```python
from build123d import *

# Parameters (mm, degrees)
EXTRUDE_1_DEPTH      = 55
CUT_EXTRUDE_START    = -5
SKETCH_2_R           = 18.75
SKETCH_2_R_2         = 14.75
CUT_EXTRUDE_1_DEPTH  = 59.016862823
EXTRUDE_3_REACH      = 65.017
EXTRUDE_3_END_RADIUS = 18.75
SKETCH_4_W           = 7
SKETCH_4_H           = 7
SKETCH_3_R           = 1.1
CUT_EXTRUDE_2_DEPTH  = 5
CUT_EXTRUDE_START_2  = -4
SKETCH_5_R           = 2.5
CUT_EXTRUDE_3_DEPTH  = 60.016862823
SKETCH_6_R           = 1.1
CUT_EXTRUDE_4_DEPTH  = 4


with BuildPart() as part:
    # ｽｹｯﾁ1 → ﾎﾞｽ - 押し出し1 (new body)
    with BuildSketch(Plane(origin=(0, 0, 0), x_dir=(1, 0, 0), z_dir=(0, 1, 0))):
        with BuildLine():
            Line((0, -21.75), (0, -14.75))
            ThreePointArc((0, -14.75), (-14.75, 0), (0, 14.75))
            Line((0, 14.75), (0, 21.75))
            ThreePointArc((0, 21.75), (-21.75, 0), (0, -21.75))
        make_face()
    extrude(amount=EXTRUDE_1_DEPTH)

    # ｽｹｯﾁ2 → ｶｯﾄ - 押し出し1 (cut, through all)
    with BuildSketch(Plane(origin=(0, 55, 0), x_dir=(1, 0, 0), z_dir=(0, 1, 0)).offset(CUT_EXTRUDE_START)):
        Circle(SKETCH_2_R)
        Circle(SKETCH_2_R_2, mode=Mode.SUBTRACT)
    extrude(amount=-CUT_EXTRUDE_1_DEPTH, mode=Mode.SUBTRACT)

    # ﾎﾞｽ - 押し出し3: up to this cylinder (the profile starts inside it)
    extrude_3_end = Plane(origin=(0, 25, 0), z_dir=(0, 1, 0)) * Cylinder(EXTRUDE_3_END_RADIUS, 193.534, mode=Mode.PRIVATE)
    # ｽｹｯﾁ4 → ﾎﾞｽ - 押し出し3 (add, up to the surface)
    with BuildSketch(Plane(origin=(0, 0, 0), x_dir=(0, 0, -1), z_dir=(1, 0, 0)), mode=Mode.PRIVATE) as extrude_3_sk1:
        with Locations((-18.25, 37.5)):
            Rectangle(SKETCH_4_W, SKETCH_4_H)
    extrude_3_tool1 = extrude(extrude_3_sk1.sketch, amount=-EXTRUDE_3_REACH, mode=Mode.PRIVATE) & extrude_3_end
    add(extrude_3_tool1.solids().sort_by_distance((0, 37.5, 18.25))[0])
    # ｽｹｯﾁ4 → ﾎﾞｽ - 押し出し3 (add, up to the surface)
    with BuildSketch(Plane(origin=(0, 0, 0), x_dir=(0, 0, -1), z_dir=(1, 0, 0)), mode=Mode.PRIVATE) as extrude_3_sk2:
        with Locations((-18.25, 12.5)):
            Rectangle(SKETCH_4_W, SKETCH_4_H)
    extrude_3_tool2 = extrude(extrude_3_sk2.sketch, amount=-EXTRUDE_3_REACH, mode=Mode.PRIVATE) & extrude_3_end
    add(extrude_3_tool2.solids().sort_by_distance((0, 12.5, 18.25))[0])
    # ｽｹｯﾁ4 → ﾎﾞｽ - 押し出し3 (add, up to the surface)
    with BuildSketch(Plane(origin=(0, 0, 0), x_dir=(0, 0, -1), z_dir=(1, 0, 0)), mode=Mode.PRIVATE) as extrude_3_sk3:
        with Locations((18.25, 12.5)):
            Rectangle(SKETCH_4_W, SKETCH_4_H)
    extrude_3_tool3 = extrude(extrude_3_sk3.sketch, amount=-EXTRUDE_3_REACH, mode=Mode.PRIVATE) & extrude_3_end
    add(extrude_3_tool3.solids().sort_by_distance((0, 12.5, -18.25))[0])
    # ｽｹｯﾁ4 → ﾎﾞｽ - 押し出し3 (add, up to the surface)
    with BuildSketch(Plane(origin=(0, 0, 0), x_dir=(0, 0, -1), z_dir=(1, 0, 0)), mode=Mode.PRIVATE) as extrude_3_sk4:
        with Locations((18.25, 37.5)):
            Rectangle(SKETCH_4_W, SKETCH_4_H)
    extrude_3_tool4 = extrude(extrude_3_sk4.sketch, amount=-EXTRUDE_3_REACH, mode=Mode.PRIVATE) & extrude_3_end
    add(extrude_3_tool4.solids().sort_by_distance((0, 37.5, -18.25))[0])

    # ｽｹｯﾁ3 → ｶｯﾄ - 押し出し2 (cut)
    with BuildSketch(Plane(origin=(0, 0, 0), x_dir=(0, 0, -1), z_dir=(1, 0, 0))):
        with Locations((-18.25, 37.5)):
            Circle(SKETCH_3_R)
        with Locations(Location((18.25, 37.5, 0), (0, 0, 180))):
            Circle(SKETCH_3_R)
        with Locations((18.25, 12.5)):
            Circle(SKETCH_3_R)
        with Locations(Location((-18.25, 12.5, 0), (0, 0, 180))):
            Circle(SKETCH_3_R)
    extrude(amount=-CUT_EXTRUDE_2_DEPTH, mode=Mode.SUBTRACT)

    # ｽｹｯﾁ5 → ｶｯﾄ - 押し出し3 (cut, through all)
    with BuildSketch(Plane(origin=(0, 0, 0), x_dir=(0, 0, -1), z_dir=(1, 0, 0)).offset(CUT_EXTRUDE_START_2)):
        with Locations((-18.25, 37.5)):
            Circle(SKETCH_5_R)
        with Locations((-18.25, 12.5)):
            Circle(SKETCH_5_R)
        with Locations((18.25, 12.5)):
            Circle(SKETCH_5_R)
        with Locations((18.25, 37.5)):
            Circle(SKETCH_5_R)
    extrude(amount=-CUT_EXTRUDE_3_DEPTH, mode=Mode.SUBTRACT)

    # ｽｹｯﾁ6 → ｶｯﾄ - 押し出し4 (cut)
    with BuildSketch(Plane(origin=(0, 55, 0), x_dir=(1, 0, 0), z_dir=(0, 1, 0))):
        with Locations(Location((-12.904698757, -12.904698757, 0), (0, 0, 270))):
            Circle(SKETCH_6_R)
        with Locations(Location((-12.904698757, 12.904698757, 0), (0, 0, 270))):
            Circle(SKETCH_6_R)
    extrude(amount=-CUT_EXTRUDE_4_DEPTH, mode=Mode.SUBTRACT)


solid = part.part
```
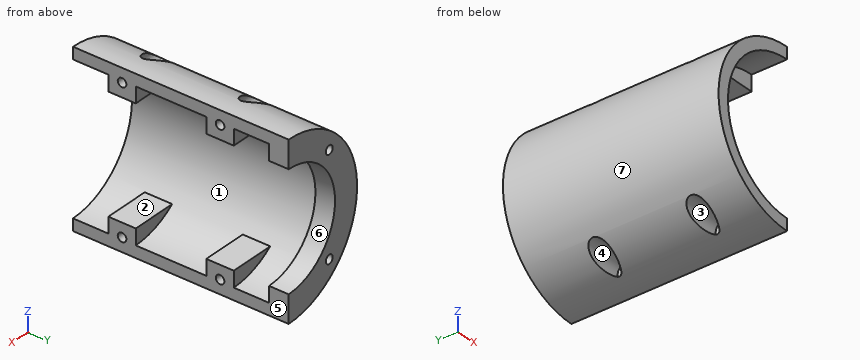
Check sheet for the modelled part. Datum: model origin and axes. Units: mm. Face numbers are marked on the shaded views. A direction names the side the tool comes from. Coordinates: 2 decimals unless noted, no trailing zeros. Write each loop counter-clockwise with the first axis right and the second up, starting at its lowest first coordinate (ties: lowest second). Pieces come first, ordered by that corner, then holes. Notation, with made-up numbers: (88, 9.5) - (128, 9.5) arc R29 ccw to (128, 39.5) - close; hole circle Ø3 at (-22, 46.5). An arc over 180 degrees is marked (long way). One line per question, with ' | ' between items.
Item 1: Sectioned sample at B-B on y = 37.5. Record the boundary of the cut face in (x, z).
Determined:
outline: (-15, -15.75) - (-4, -15.75) - (-4, -17.15) - (0, -17.15) - (0, -14.75) - (-11.58, -14.75) arc R18.75 cw to (-11.58, 14.75) - (0, 14.75) - (0, 17.15) - (-4, 17.15) - (-4, 15.75) - (-15, 15.75) arc R21.75 ccw to start; (-6.52, -20.75) arc R21.75 ccw to (0, -21.75) - (0, -19.35) - (-4, -19.35) - (-4, -20.75) - close; (-6.52, 20.75) - (-4, 20.75) - (-4, 19.35) - (0, 19.35) - (0, 21.75) arc R21.75 ccw to start
Item 2: Access from +Z, -Z, +X, -X, +Y, -Y to the whole of each face (thin tool, end or side, straight path). Record for the marked faces 1, 2 and 3.
Determined:
face 1: +X | face 2: +X, -Y | face 3: -X
Item 3: Gauge pin test, flat ends, axial feed: P1, Ø1.5, axis at x = -14.5, z = -2, coming from the -Y side; P2, Ø3, axis at x = -12.5, y = 32.5, coming from the +Z side; P3, Ø2, axis at y = 36, z = -4.5, coming from the +X side. Record the tip position at first contact, or that the pin passes through.
Determined:
P1: stops at y = 50 | P2: stops at z = 18.76 | P3: stops at x = -17.93
Item 4: Thickness scan on line 1 (Y direction, x = -1.15, z = -18.25); line 2 (Y direction, x = -6.25, z = 18.25); line 3 (Z direction, x = -5.25, y = 37.5). Record the ranges inside material, lowest first. Write a range as [from, to].
Determined:
line 1: y = [9, 11.4], [13.6, 16], [34, 36.4], [38.6, 41], [50, 55] | line 2: y = [0, 10], [15, 35], [40, 55] | line 3: z = [-21.11, -20.75], [-15.75, -14.75], [14.75, 15.75], [20.75, 21.11]
Item 5: Sectioned sample at A-A on x = -1.5. Give the number of separate pieces and of enclosed holes in the cut face, plus the area to 3 significant figures.
Determined:
separate pieces: 2 | enclosed holes: 4 | area: 466 mm2
Item 6: Sectioned sample at C-C on z = 0. Record the boundary of the cut face in (x, y), plus the area to 3 significant figures.
Determined:
outline: (-21.75, 0) - (-18.75, 0) - (-18.75, 50) - (-14.75, 50) - (-14.75, 55) - (-21.75, 55) - close | area: 185 mm2
Item 7: Sectioned sample at D-D on x = -18. Record the boundary of the cut face in (y, z).
Determined:
outline: (0, -12.21) - (55, -12.21) - (55, 12.21) - (0, 12.21) - (0, 5.25) - (50, 5.25) - (50, -5.25) - (0, -5.25) - close
Item 8: Mould release check, pull along Z, two halves, no side actions. Record for the marked faces 4, 5, 6 and 7: pulls with the +Z half, pulls with the -Z half, needs draft (parallel to the pull), parting line crosses it, or undercut.
Determined:
face 4: undercut | face 5: needs draft | face 6: undercut | face 7: parting line crosses it
